Geometry: see drawing. Coordinates: mm, zero at the bounding-box minimum. Give positions to 0.01 mm unless a question says otherwise; leave off trailing zeros. Loops run counter-clockwise (first coordinate to the right, second up) from the corner with the lowest first, then second, coordinate; pieces in that order, holes last. Notation, with made-up numbers: (63.25, 37.5) -> (116.25, 37.5) arc R11 cw to (116.25, 58.5) -> close; hole circle Ø7 at (72.5, -20). An arc over 180 degrees is marked (long way). Use CSV: the item, a comma, the result in double quotes.
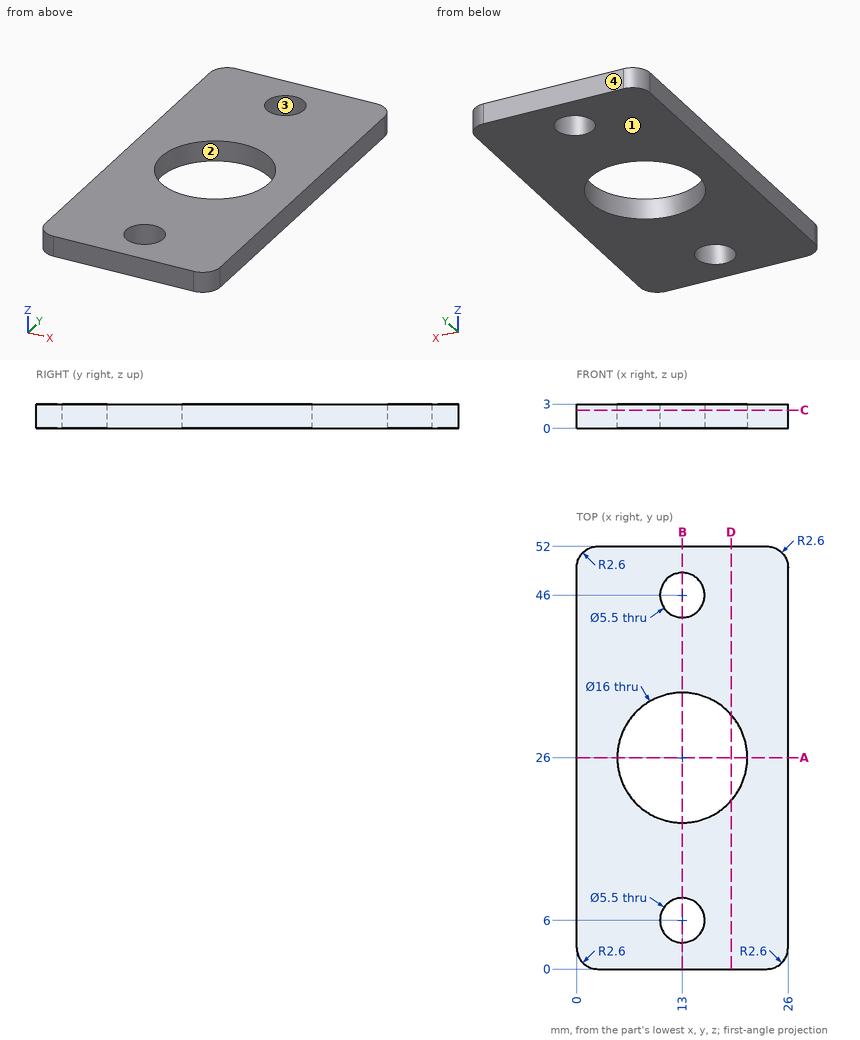
1) Contact query for a flat-ended pin moving along its axis: pin 1 (4.5 mm diameter, centred on x = 13, y = 6, fed in from -Z). Output: stop coordinate, or through.
From the geometry:
pin 1,"passes through"
2) Section query D-D (x = 19). Return loops of the section in (y, z).
From the geometry:
outline,"(0, 0) -> (20.71, 0) -> (20.71, 3) -> (0, 3) -> close; (31.29, 0) -> (52, 0) -> (52, 3) -> (31.29, 3) -> close"
3) Section query B-B (x = 13). Return loops of the section in (y, z), then the cut area to 3 significant figures.
From the geometry:
outline,"(0, 0) -> (3.25, 0) -> (3.25, 3) -> (0, 3) -> close; (8.75, 0) -> (18, 0) -> (18, 3) -> (8.75, 3) -> close; (34, 0) -> (43.25, 0) -> (43.25, 3) -> (34, 3) -> close; (48.75, 0) -> (52, 0) -> (52, 3) -> (48.75, 3) -> close"
area,"75.0 mm^2"
4) Mould query, pull axis Y, two halves, no side actions, for the marked faces 1, 2, 3 and 4. Classes: pulls with the +Y half, pulls with the -Y half, needs draft (parallel to the pull), parting line crosses it, or undercut.
From the geometry:
face 1,"needs draft"
face 2,"undercut"
face 3,"undercut"
face 4,"pulls with the +Y half"
5) Ray query, line 1 (Y direction, x = 13, z = 1.35); line 2 (Y direction, x = 12, z = 1.3); line 3 (Y direction, x = 16.75, z = 1.2). Return the intervals inside material, ascending.
From the geometry:
line 1,"y = 0 to 3.25, 8.75 to 18, 34 to 43.25, 48.75 to 52"
line 2,"y = 0 to 3.44, 8.56 to 18.06, 33.94 to 43.44, 48.56 to 52"
line 3,"y = 0 to 18.93, 33.07 to 52"
6) Section query A-A (y = 26). Return loops of the section in (x, z), then the cut area to 3 significant figures.
From the geometry:
outline,"(0, 0) -> (5, 0) -> (5, 3) -> (0, 3) -> close; (21, 0) -> (26, 0) -> (26, 3) -> (21, 3) -> close"
area,"30.0 mm^2"
7) Section query C-C (z = 2.25). Return loops of the section in (x, y).
From the geometry:
outline,"(0, 2.6) arc R2.6 ccw to (2.6, 0) -> (23.4, 0) arc R2.6 ccw to (26, 2.6) -> (26, 49.4) arc R2.6 ccw to (23.4, 52) -> (2.6, 52) arc R2.6 ccw to (0, 49.4) -> close; hole circle Ø16 at (13, 26); hole circle Ø5.5 at (13, 6); hole circle Ø5.5 at (13, 46)"
